The listing builds one solid part. Answer for the finished solid, in the listing's coordinates (mm). A direction names the side the tool comes from. Round coordinates to 2 decimals unless told otherwise and drop trailing zeros. Write each loop counter-clockwise with the first axis right and the second up, starting at its lowest first coordinate (ties: lowest second). Pieces come first, ordered by that corner, then holes.
Item 1: A tool of negligible diameter and unlimited length cuts with its end or side. For faces 4 (the face through (-11, -15, 68)), 5 (the face through (-11, -19, 62)), 6 (the face through (-39, -10, 25)), from which of +Z, -Z, +X, -X, +Y, -Y can it reach the whole face along a straight path? Write none if from no direction.
Item 2: Each of these flat-tipped pins is pushed along its axis until it touches: pin 1 (17.5 mm diameter, centred on y = -10.5, z = 30.5, fed in from -X); pin 2 (8 mm diameter, centred on x = -4.5, y = -17, fed in from +Z); pin 3 (18.5 mm diameter, centred on x = 11, z = 29.5, fed in from -Y); pin 4 (5 mm diameter, centred on x = -24.5, z = 25.5, fed in from -Y). Where does it stop, or does it pass through?
Item 3: Find section B-B on x = 13. Give the vertices of the cut face in (y, z).
Item 4: Find the intervals of material crossed by probe 1 along X at (y, z) = (-40, 67) (3 decimals); probe 2 along X at (y, z) = (-16, 61); probe 3 along Z at (x, y) = (13, -14.5), in increasing order.
Item 5: Find section C-C on y = -23. Give the vertices of the cut face in (x, z), then the cut area to 3 significant figures.
Item 6: Find section A-A on z = 13. Give the vertices of the cut face in (x, y).
Item 7: For a pull along Z with two mould halves and no side action, classify faces 1 (the face through (17, -10, 20)), 2 (the face through (22.1, -40.98, 74.14)), 3 (the face through (3, -39, 67)) as +Z half, -Z half, draft (parallel to the pull), parting line (faces both ways), or undercut.
Item 8: Find section D-D on y = -13. Give the vertices of the cut face in (x, z), then the cut area to 3 significant figures.
```python
from build123d import *

# Parameters (mm, degrees)
BOSS_EXTRUDE1_DEPTH = 10
SKETCH2_W           = 66.5
SKETCH2_H           = 6
BOSS_EXTRUDE2_DEPTH = 42
BOSS_EXTRUDE3_DEPTH = 10
SKETCH3_R           = 20.035
CUT_EXTRUDE2_DEPTH  = 10
FILLET1_R           = 12
SKETCH7_W           = 66.5
SKETCH7_H           = 4
BOSS_EXTRUDE4_DEPTH = 7
SKETCH8_R           = 3.025
CUT_EXTRUDE3_DEPTH  = 3
FILLET2_R           = 12
FILLET3_R           = 10
FILLET4_R           = 3
FILLET5_R           = 3


with BuildPart() as part:
    # Sketch1 → Boss-Extrude1 (new body)
    with BuildSketch(Plane(origin=(0, 0, 0), x_dir=(1, 0, 0), z_dir=(0, 1, 0))):
        Polygon((0, 0), (-43.5, 0), (-43.5, -68), (23, -68), (23, 0), align=None)
    extrude(amount=BOSS_EXTRUDE1_DEPTH)

    # Sketch2 → Boss-Extrude2 (add)
    with BuildSketch(Plane.XZ):
        with Locations((-10.25, 65)):
            Rectangle(SKETCH2_W, SKETCH2_H)
    extrude(amount=BOSS_EXTRUDE2_DEPTH)

    # Sketch4 → Boss-Extrude3 (add)
    with BuildSketch(Plane.XZ):
        Polygon((-43.5, 62), (-36, 62), (-36, 7.5), (15.5, 7.5), (15.5, 62), (23, 62), (23, 0), (-43.5, 0), align=None)
    extrude(amount=BOSS_EXTRUDE3_DEPTH)

    # Sketch3 → Cut-Extrude2 (cut)
    with BuildSketch(Plane(origin=(0, 0, 0), x_dir=(-1, 0, 0), z_dir=(0, 0, -1))):
        with Locations((16, -22)):
            Circle(SKETCH3_R)
    extrude(amount=-CUT_EXTRUDE2_DEPTH, mode=Mode.SUBTRACT)

    # Fillet1
    fillet1_edges = [part.edges().sort_by_distance(p)[0] for p in [
        (19.25, -10, 62),
        (-39.75, -10, 62),
    ]]
    fillet(fillet1_edges, radius=FILLET1_R)

    # Sketch7 → Boss-Extrude4 (add)
    with BuildSketch(Plane.XY.offset(68)):
        with Locations((-10.25, -40)):
            Rectangle(SKETCH7_W, SKETCH7_H)
    extrude(amount=BOSS_EXTRUDE4_DEPTH)

    # Sketch8 → Cut-Extrude3 (cut)
    with BuildSketch(Plane.XZ.offset(42)):
        with Locations(Location((-28.5, 67, 0), (0, 0, 270))):
            Circle(SKETCH8_R)
        with Locations(Location((3, 67, 0), (0, 0, 270))):
            Circle(SKETCH8_R)
    extrude(amount=-CUT_EXTRUDE3_DEPTH, mode=Mode.SUBTRACT)

    # Fillet2
    fillet2_edges = [part.edges().sort_by_distance(p)[0] for p in [
        (-10.25, 10, 68),
    ]]
    fillet(fillet2_edges, radius=FILLET2_R)

    # Fillet3
    # the kernel refuses this fillet: 10 mm, written as the material it adds along each edge
    with BuildSketch(Plane(origin=(23, -38, 68), x_dir=(0, 1, 0), z_dir=(-1, 0, 0))) as fillet3_piece_1:
        with BuildLine():
            CenterArc((9.539392014, -10), FILLET3_R, 90, 72.542396876)
            Line((0, -7), (-0.19078784, -6.94))
            ThreePointArc((-0.19078784, -6.94), (-0.2, -3.5), (-0.2, 0))
            Line((-0.2, 0), (0, 0.2))
            Line((0, 0.2), (9.539392014, 0.2))
            Line((9.539392014, 0.2), (9.539392014, 0))
        make_face()
    extrude(amount=66.5)

    # Fillet4
    # the kernel refuses this fillet: 3 mm, written as the material it takes off along each edge
    with BuildSketch(Plane(origin=(-51, -42, 62), x_dir=(0, 0, 1), z_dir=(1, 0, 0))) as fillet4_piece_1:
        with BuildLine():
            CenterArc((FILLET4_R, -FILLET4_R), FILLET4_R, 90, 90)
            Line((0, -FILLET4_R), (0, 0))
            Line((0, 0), (FILLET4_R, 0))
        make_face()
    extrude(amount=81.5, mode=Mode.SUBTRACT)

    # Fillet5
    fillet5_edges = [part.edges().sort_by_distance(p)[0] for p in [
        (23, 10, 28),
        (23, -15.230303993, 68),
        (23, 6.485281374, 64.485281374),
        (-43.5, -15.230303993, 68),
        (-43.5, 6.485281374, 64.485281374),
        (-43.5, -34.376687769, 69.937742252),
        (23, -34.376687769, 69.937742252),
        (-43.5, 10, 28),
        (-10.25, 10, 0),
        (-43.5, -40, 75),
        (23, -40, 75),
        (23, 0, 0),
        (-10.25, -38, 75),
        (-43.5, 0, 0),
    ]]
    fillet(fillet5_edges, radius=FILLET5_R)


solid = part.part
```
Check values:
1. face 4: +Z, +X, -X, +Y
1. face 5: -Y
1. face 6: -Z, +X, -X, -Y
2. pin 1: stops at x = -43.5
2. pin 2: stops at z = 68
2. pin 3: stops at y = -10
2. pin 4: stops at y = 0
3. outline: (-42, 65) arc R3 ccw to (-39, 62) - (0, 62) - (0, 7.5) - (-10, 7.5) - (-10, 0) - (7, 0) arc R3 ccw to (10, 3) - (10, 56) arc R12 ccw to (-2, 68) - (-28.46, 68) arc R10 cw to (-37.33, 73.38) arc R3 ccw to (-39.99, 75) - (-42, 75) - close
4. probe 1: x = -43.5 to -31.525, -25.475 to -0.025, 6.025 to 23
4. probe 2: x = -43.5 to -36, 15.5 to 23
4. probe 3: z = 62 to 68
5. outline: (-43.5, 62) - (23, 62) - (23, 65) arc R3 ccw to (20, 68) - (-40.5, 68) arc R3 ccw to (-43.5, 65) - close
5. area: 395 mm2
6. outline: (-43.5, -10) - (-36, -10) - (-36, 0) - (15.5, 0) - (15.5, -10) - (23, -10) - (23, 7) arc R3 ccw to (20, 10) - (-40.5, 10) arc R3 ccw to (-43.5, 7) - close
7. face 1: draft
7. face 2: +Z half
7. face 3: undercut
8. outline: (-43.5, 57.94) - (-36, 57.94) - (-36, 62) - (15.5, 62) - (15.5, 57.94) - (23, 57.94) - (23, 65) arc R3 ccw to (20, 68) - (-40.5, 68) arc R3 ccw to (-43.5, 65) - close
8. area: 456 mm2
